```python
from build123d import *

# Parameters (mm, degrees)
F0_W      = 101.6
F0_H      = 50.8
F1_DEPTH  = 6.35
F2_W      = 25.4
F2_H      = 50.8
F3_DEPTH  = 31.75
F4_R      = 9.525
F5_DEPTH  = 50.801
F6_W      = 76.2
F6_H      = 6.35
F7_DEPTH  = 6.35
F8_DEPTH  = 25.4
F9_SIZE2  = 25.3483661935
F9_SIZE   = 76.2
F10_R     = 3.175
F11_DEPTH = 25.4
F12_R     = 3.175
F13_DEPTH = 25.4


with BuildPart() as f1:
    # F0 (on Top) → F1 (new body)
    with BuildSketch(Plane.XY):
        with Locations((-14.6277205467, -8.5982844889)):
            Rectangle(F0_W, F0_H)
    extrude(amount=F1_DEPTH)

    # F2 (on face) → F3 (join)
    with BuildSketch(Plane.XY.offset(6.35)):
        with Locations((-52.7277205467, -8.5982844889)):
            Rectangle(F2_W, F2_H)
    extrude(amount=F3_DEPTH)

    # F4 (on face) → F5 (cut, through all)
    with BuildSketch(Plane.XZ.offset(33.9982844889)):
        with Locations((-52.7277205467, 25.4)):
            Circle(F4_R)
    extrude(amount=-F5_DEPTH, mode=Mode.SUBTRACT)

    # F6 (on face) → F7 (join)
    with BuildSketch(Plane.XY.offset(6.35)):
        with Locations((-1.9277205467, -8.5982844889)):
            Rectangle(F6_W, F6_H)
    extrude(amount=F7_DEPTH)

    # F8 (add): a face of the model
    f8_faces = [f1.faces().sort_by_distance(p)[0] for p in [
        (-1.9277205467, -8.5982844889, 12.7),
    ]]
    extrude(f8_faces, amount=F8_DEPTH)

    # F9
    f9_edges = [f1.edges().sort_by_distance(p)[0] for p in [
        (36.172279, -8.598284, 38.1),
    ]]
    f9_side = f1.faces().sort_by_distance((-38.873175, -8.598284, 38.1))[0]
    chamfer(f9_edges, length=F9_SIZE, length2=F9_SIZE2, reference=f9_side)

    # F10 (on face) → F11 (cut)
    with BuildSketch(Plane.XY.offset(6.35)):
        with Locations((25.0597794533, 5.6892155111)):
            Circle(F10_R)
        with Locations((-28.9152205467, 5.6892155111)):
            Circle(F10_R)
    extrude(amount=-F11_DEPTH, mode=Mode.SUBTRACT)

    # F12 (on face) → F13 (cut)
    with BuildSketch(Plane.XY.offset(6.35)):
        with Locations((-28.9152205467, -22.8857844889)):
            Circle(F12_R)
        with Locations((25.0597794533, -22.8857844889)):
            Circle(F12_R)
    extrude(amount=-F13_DEPTH, mode=Mode.SUBTRACT)


solid = f1.part
```
Can you work these out from the model? Positions are in its coordinate system, mm. A direction names the side the tool comes from. Round coordinates to 2 decimals unless told otherwise and drop trailing zeros. Loops run counter-clockwise (first coordinate to the right, second up) from the corner with the lowest first, then second, coordinate; pieces in that order, holes last. Notation, with made-up numbers: M 6.25,69.25 L 21.25,69.25 A8 cw 21.25,78.25 Z; hole C 29,55 d4. An arc over 180 degrees is marked long. Answer as a JSON object with one key per item and string values. Group by question number.
Q1. Will these pins go through, and if not, where does the flat tip stop? pin 1 (2 mm diameter, centred on x = -35.5, y = -17, fed in from +Z); pin 2 (16 mm diameter, centred on x = -8.5, z = 25.5, fed in from +Y); pin 3 (18 mm diameter, centred on y = -23, z = 21.5, fed in from +X).
Q2. We'd pull the mould along X, two halves only. Please class faces 1 (the flat face through (-65.428, -9, 19)), 2 (the cylindrical face through (27.993, -24.102, 3.219)), 3 (the flat face through (-2, -23, 6.35)), 4 (the cylindrical face through (-25.98, -24.1, 3.22)): +X half, -X half, draft (parallel to the pull), parting line (faces both ways), or undercut.
Q3. Imagine slicing it at B-B, the plane z = 32. Please give me the cut outline in (x, y), then the cut area to 3 significant figures.
Q4. Imagine slicing it at C-C, the plane y = -7. Please give me the cut outline in (x, z) (3 decimals), then the cut area to 3 significant figures.
Q5. On a 3-axis mill with a long thin cutter (end or side, diameter ignored), from which of +Z, -Z, +X, -X, +Y, -Y can I reach the whole of each face in a straight line? I mean faces 5 (the flat face through (-40.028, 6, 22)), 6 (the flat face through (-40.028, -23, 22)), 7 (the cylindrical face through (27.99, 4.47, 3.22)). Say none if no direction works.
Q6. Please list where these lines run through material, in increasing order: L1, parallel to X at y = -23, z = 25; L2, parallel to Z at x = -23, y = -16; L3, parallel to X at y = -15.5, z = 10.5.
Q7. Imagine slicing it at A-A, the plane y = -29.5. Please give me the cut outline in (x, z) (3 decimals), then the cut area to 3 significant figures.
Q8. Imagine slicing it at D-D, the plane x = -14. Please give me the cut outline in (y, z), then the cut area to 3 significant figures.
Findings:
{
 "1": {"pin 1": "stops at z = 6.35", "pin 2": "stops at y = -5.42", "pin 3": "stops at x = -40.03"},
 "2": {"face 1": "-X half", "face 2": "undercut", "face 3": "draft", "face 4": "undercut"},
 "3": {"outline": "M -65.43,-34 L -59.6,-34 L -59.6,16.8 L -65.43,16.8 Z; M -45.86,-34 L -40.03,-34 L -40.03,-11.77 L -21.69,-11.77 L -21.69,-5.42 L -40.03,-5.42 L -40.03,16.8 L -45.86,16.8 Z", "area": "709 mm2"},
 "4": {"outline": "M -65.428,0 L 36.172,0 L 36.172,12.752 L -40.028,38.1 L -65.428,38.1 Z; hole C -52.728,25.4 d19.05", "area": "2,620 mm2"},
 "5": {"face 5": "+Z, +X, +Y", "face 6": "+Z, +X, -Y", "face 7": "+Z, -Z"},
 "6": {"L1": "x = -65.43 to -62.24, -43.21 to -40.03", "L2": "z = 0 to 6.35", "L3": "x = -65.43 to -40.03"},
 "7": {"outline": "M -65.428,0 L 36.172,0 L 36.172,6.35 L -40.028,6.35 L -40.028,38.1 L -65.428,38.1 Z; hole C -52.728,25.4 d19.05", "area": "1,170 mm2"},
 "8": {"outline": "M -34,0 L 16.8,0 L 16.8,6.35 L -5.42,6.35 L -5.42,29.44 L -11.77,29.44 L -11.77,6.35 L -34,6.35 Z", "area": "469 mm2"}
}
